Input: part model. Units: mm. Frame: model coordinates. A direction names the side the tool comes from. Round coordinates to 2 decimals unless told otherwise and drop trailing zeros. Loops run counter-clockwise (first coordinate to the right, second up) from the corner with the lowest first, then second, coordinate; pieces in that order, holes last. Notation, with made-up numbers: (79.5, 9.25) - (131.5, 9.25) arc R13 ccw to (131.5, 17.25) - close; hole circle Ø4 at (16, 3.25). An arc over 180 degrees is marked (long way). One line per question, with ' | ' between items. Start each with the question number.
from build123d import *

# Parameters (mm, degrees)
SKETCH1_W                = 100
SKETCH1_H                = 110
BOSS_EXTRUDE1_DEPTH      = 6.86
BOSS_EXTRUDE2_DEPTH      = 6.86
CUT_EXTRUDE1_DEPTH       = 84.419927529
CUT_EXTRUDE1_DEPTH_BACK  = 84.419927529
CUT_EXTRUDE5_DEPTH       = 84.419927529
CUT_EXTRUDE6_DEPTH       = 84.419927529
SKETCH7_W                = 42
SKETCH7_H                = 3.55
CUT_EXTRUDE7_DEPTH       = 84.419927529
SKETCH8_W                = 5
SKETCH8_H                = 7.62
CUT_EXTRUDE8_DEPTH       = 84.419927529
CUT_EXTRUDE9_DEPTH       = 84.419927529
LPATTERN1_COUNT          = 2
LPATTERN1_PITCH          = 49.4
SKETCH15_W               = 6.5
SKETCH15_H               = 9.5
BOSS_EXTRUDE3_DEPTH      = 6.86
CUT_EXTRUDE14_START      = -6.86
CUT_EXTRUDE14_DEPTH      = 6.86
BOSS_EXTRUDE4_DEPTH      = 6.86
FILLET3_R                = 5
FILLET4_R                = 7
CUT_EXTRUDE11_DEPTH      = 84.419927529
BOSS_EXTRUDE5_DEPTH      = 6.86
BOSS_EXTRUDE6_DEPTH      = 6.86
CUT_EXTRUDE12_DEPTH      = 84.419927529
CUT_EXTRUDE12_DEPTH_BACK = 84.419927529
SKETCH22_R               = 1
CUT_EXTRUDE13_DEPTH      = 84.419927529
CUT_EXTRUDE15_DEPTH      = 84.419927529
CUT_EXTRUDE15_DEPTH_BACK = 84.419927529
CUT_EXTRUDE16_DEPTH      = 84.419927529
CUT_EXTRUDE16_DEPTH_BACK = 84.419927529
FILLET2_R                = 1
BOSS_EXTRUDE8_START      = -6.86
BOSS_EXTRUDE8_DEPTH      = 6.86
CUT_EXTRUDE19_START      = -10
CUT_EXTRUDE19_DEPTH      = 10
SKETCH28_W               = 6.86
SKETCH28_H               = 9.5
SKETCH28_H_2             = 35
BOSS_EXTRUDE9_DEPTH      = 0.4
BOSS_EXTRUDE10_REACH     = 81.915
SKETCH29_W               = 6.86
SKETCH29_H               = 0.5
BOSS_EXTRUDE11_DEPTH     = 6.86


# Read off the part's stored shape, not the designer's step: Cut-Extrude14
with BuildPart() as part:
    # Sketch1 → Boss-Extrude1 (new body)
    with BuildSketch(Plane.XY):
        Rectangle(SKETCH1_W, SKETCH1_H)
    extrude(amount=BOSS_EXTRUDE1_DEPTH)

    # Sketch14 → Boss-Extrude2 (add)
    with BuildSketch(Plane.XY.offset(6.86)):
        with BuildLine():
            Line((-50, 44), (-56.9, 44))
            Line((-56.9, 44), (-57.252653961, 46))
            Line((-57.252653961, 46), (-60.252653961, 46))
            ThreePointArc((-60.252653961, 46), (-62.140394827, 27.177051725), (-56.9, 9))
            Line((-56.9, 9), (-50, 9))
            Line((-50, 9), (-50, 44))
        make_face()
    extrude(amount=-BOSS_EXTRUDE2_DEPTH)

    # Sketch9 → Cut-Extrude1 (cut, two sides: drawn at the far end of the back side and taken through both)
    with BuildSketch(Plane.XY.offset(6.86).offset(-CUT_EXTRUDE1_DEPTH_BACK)):
        Polygon((-202.691345573, 326.397371639), (-46, 55), (2.5, -29.004464167), (-49.825975731, -59.214880341), (-321.22334737, -215.906225914), (291.08659924, -349.739606366), (409.618601037, 192.563991188), align=None)
    extrude(amount=CUT_EXTRUDE1_DEPTH + CUT_EXTRUDE1_DEPTH_BACK, mode=Mode.SUBTRACT)

    # Sketch11 → Cut-Extrude5 (cut, through all)
    with BuildSketch(Plane.XY.offset(6.86)):
        Polygon((-35.90593882, 37.516573181), (-8.20593882, -10.461234188), (-15.13414205, -14.461234188), (-42.83414205, 33.516573181), align=None)
    extrude(amount=-CUT_EXTRUDE5_DEPTH, mode=Mode.SUBTRACT)

    # Sketch12 → Cut-Extrude6 (cut, through all)
    with BuildSketch(Plane.XY.offset(6.86)):
        Polygon((-18.88414205, -7.96604366), (-21.534179786, -9.49604366), (-35.534179786, 14.752667646), (-32.88414205, 16.282667646), align=None)
    extrude(amount=-CUT_EXTRUDE6_DEPTH, mode=Mode.SUBTRACT)

    # Sketch7 → Cut-Extrude7 (cut, through all)
    with BuildSketch(Plane.XY.offset(6.86)):
        with Locations((-50, -34)):
            Rectangle(SKETCH7_W, SKETCH7_H)
    extrude(amount=-CUT_EXTRUDE7_DEPTH, mode=Mode.SUBTRACT)

    # Sketch8 → Cut-Extrude8 (cut, through all)
    with BuildSketch(Plane.XY.offset(6.86)):
        with Locations((-36.5, -34)):
            Rectangle(SKETCH8_W, SKETCH8_H)
    extrude(amount=-CUT_EXTRUDE8_DEPTH, mode=Mode.SUBTRACT)

    # Sketch13 → Cut-Extrude9 (cut, through all)
    with BuildSketch(Plane.XY.offset(6.86)):
        Polygon((-41.88414205, 31.871124914), (-40.78414205, 29.965869026), (-48.578370684, 25.465869026), (-48.048870684, 24.548748123), (-49.478678626, 23.723248123), (-50.008178626, 24.640369026), (-52.908497703, 22.965869026), (-54.008497703, 24.871124914), (-51.108178626, 26.545624914), (-51.637678626, 27.462745817), (-50.207870684, 28.288245817), (-49.678370684, 27.371124914), align=None)
        Polygon((-39.45593882, 43.665353548), (-38.35593882, 41.76009766), (-46.150167454, 37.26009766), (-45.620667454, 36.342976757), (-47.050475396, 35.517476757), (-47.579975396, 36.43459766), (-50.480294473, 34.76009766), (-51.580294473, 36.665353548), (-48.679975396, 38.339853548), (-49.209475396, 39.256974451), (-47.779667454, 40.082474451), (-47.250167454, 39.165353548), align=None)
        Polygon((-18.443009001, -24.930108514), (-11.443009001, -37.054464167), (-9.537753113, -35.954464167), (-16.537753113, -23.830108514), align=None)
    cut_extrude9 = extrude(amount=-CUT_EXTRUDE9_DEPTH, mode=Mode.SUBTRACT)

    # LPattern1: Cut-Extrude9 ×2
    with Locations(*[Vector(0.49999999999999345, -0.8660254037844425, 0) * (i * LPATTERN1_PITCH) for i in range(1, LPATTERN1_COUNT)]):
        add(cut_extrude9, mode=Mode.SUBTRACT)

    # Sketch15 → Boss-Extrude3 (add)
    with BuildSketch(Plane.XY.offset(6.86)):
        with Locations((-53.25, -19.75)):
            Rectangle(SKETCH15_W, SKETCH15_H)
    extrude(amount=-BOSS_EXTRUDE3_DEPTH)

    # Cut-Extrude14 outline → Cut-Extrude14 (cut)
    with BuildSketch(Plane.XY.offset(6.86).offset(CUT_EXTRUDE14_START)):
        Polygon((-56.5, -15), (-56.5, -16.500643242), (-50, -15), align=None)
    extrude(amount=CUT_EXTRUDE14_DEPTH, mode=Mode.SUBTRACT)

    # Sketch16 → Boss-Extrude4 (add)
    with BuildSketch(Plane.XY.offset(6.86)):
        Polygon((-35.605117767, -51.004464167), (-34.105117767, -53.602540378), (-36.525588833, -55), (-42.525588833, -55), (-44.558274136, -51.479285778), align=None)
    extrude(amount=-BOSS_EXTRUDE4_DEPTH)

    # Fillet3
    fillet3_edges = [part.edges().sort_by_distance(p)[0] for p in [
        (2.5, -29.004464167, 3.43),
    ]]
    fillet(fillet3_edges, radius=FILLET3_R)

    # Fillet4
    fillet4_edges = [part.edges().sort_by_distance(p)[0] for p in [
        (-56.9, 9, 3.43),
    ]]
    fillet(fillet4_edges, radius=FILLET4_R)

    # Sketch18 → Cut-Extrude11 (cut, through all)
    with BuildSketch(Plane.XY.offset(6.86)):
        Polygon((-17.686495929, -28.360427591), (-13.945266185, -26.200427591), (-13.119766185, -27.630235533), (-16.860995929, -29.790235533), align=None)
    extrude(amount=-CUT_EXTRUDE11_DEPTH, mode=Mode.SUBTRACT)

    # Sketch19 → Boss-Extrude5 (add)
    with BuildSketch(Plane.XY.offset(6.86)):
        Polygon((-24.334179786, -4.646301399), (-23.234179786, -6.551557287), (-25.780294473, -8.021557287), (-26.880294473, -6.116301399), align=None)
    extrude(amount=-BOSS_EXTRUDE5_DEPTH)

    # Sketch20 → Boss-Extrude6 (add)
    with BuildSketch(Plane.XY.offset(6.86)):
        Polygon((-32.88414205, 16.282667646), (-18.88414205, -7.96604366), (-23.822038778, -10.816939665), (-37.822038778, 13.431771641), align=None)
    extrude(amount=-BOSS_EXTRUDE6_DEPTH)

    # Sketch21 → Cut-Extrude12 (cut, two sides: drawn at the far end of the back side and taken through both)
    with BuildSketch(Plane.XY.offset(6.86).offset(-CUT_EXTRUDE12_DEPTH_BACK)):
        Polygon((-50, 55), (-50, 44), (-48.060403212, 55), align=None)
    extrude(amount=CUT_EXTRUDE12_DEPTH + CUT_EXTRUDE12_DEPTH_BACK, mode=Mode.SUBTRACT)

    # Sketch22 → Cut-Extrude13 (cut, through all)
    with BuildSketch(Plane.XY.offset(6.86)):
        with Locations((-38, -5)):
            Circle(SKETCH22_R)
    extrude(amount=-CUT_EXTRUDE13_DEPTH, mode=Mode.SUBTRACT)

    # Sketch24 → Cut-Extrude15 (cut, two sides: drawn at the far end of the back side and taken through both)
    with BuildSketch(Plane.XY.offset(6.86).offset(-CUT_EXTRUDE15_DEPTH_BACK)):
        Polygon((207.425051562, 16.452548282), (-35.605117767, -51.004464167), (-50, -55), (-293.030169328, -122.457012449), (-158.11614443, -608.517351106), (342.33907646, -469.607790375), align=None)
    extrude(amount=CUT_EXTRUDE15_DEPTH + CUT_EXTRUDE15_DEPTH_BACK, mode=Mode.SUBTRACT)

    # Sketch26 → Cut-Extrude16 (cut, two sides: drawn at the far end of the back side and taken through both)
    with BuildSketch(Plane.XY.offset(6.86).offset(-CUT_EXTRUDE16_DEPTH_BACK)):
        Polygon((209.546353054, 0.01089), (-35.605117767, -51.004464167), (-50, -54), (-295.15147082, -105.015354167), (-193.120762486, -595.318295807), (311.577061387, -490.29205164), align=None)
    extrude(amount=CUT_EXTRUDE16_DEPTH + CUT_EXTRUDE16_DEPTH_BACK, mode=Mode.SUBTRACT)

    # Fillet2
    fillet2_edges = [part.edges().sort_by_distance(p)[0] for p in [
        (-60.252653961, 46, 3.43),
        (-56.5, -24.5, 3.43),
        (-56.5, -16.500643242, 3.43),
        (-50, -54, 3.43),
    ]]
    fillet(fillet2_edges, radius=FILLET2_R)

    # Sketch27 → Boss-Extrude8 (add)
    with BuildSketch(Plane.XY.offset(6.86).offset(BOSS_EXTRUDE8_START)):
        with BuildLine():
            Line((-55.724951054, -16.321709094), (-50, -15))
            Line((-50, -15), (-56.5, -15))
            Line((-56.5, -15), (-56.5, -17.296079159))
            ThreePointArc((-56.5, -17.296079159), (-56.282608157, -16.673564522), (-55.724951054, -16.321709094))
        make_face()
        with BuildLine():
            ThreePointArc((-52.380008746, 9), (-54.54635817, 9.343654894), (-56.5, 10.340877094))
            Line((-56.5, 10.340877094), (-56.5, 9))
            Line((-56.5, 9), (-52.380008746, 9))
        make_face()
        with BuildLine():
            Line((-56.5, -24.5), (-55.5, -24.5))
            ThreePointArc((-55.5, -24.5), (-56.207106781, -24.207106781), (-56.5, -23.5))
            Line((-56.5, -23.5), (-56.5, -24.5))
        make_face()
    extrude(amount=BOSS_EXTRUDE8_DEPTH)

    # Sketch27<5> → Cut-Extrude19 (cut)
    with BuildSketch(Plane.XY.offset(6.86).offset(CUT_EXTRUDE19_START)):
        with BuildLine():
            Line((-56.5, 10.340877094), (-56.5, 44))
            Line((-56.5, 44), (-56.9, 44))
            Line((-56.9, 44), (-57.252653961, 46))
            Line((-57.252653961, 46), (-59.50182182, 46))
            ThreePointArc((-59.50182182, 46), (-60.105291207, 45.797386167), (-60.464218102, 45.271649399))
            ThreePointArc((-60.464218102, 45.271649399), (-62.283923616, 29.230647449), (-58.897432775, 13.445947531))
            ThreePointArc((-58.897432775, 13.445947531), (-57.920678072, 11.722035132), (-56.5, 10.340877094))
        make_face()
    extrude(amount=CUT_EXTRUDE19_DEPTH, mode=Mode.SUBTRACT)

    # Sketch28 → Boss-Extrude9 (add)
    with BuildSketch(Plane.ZY.offset(56.5)):
        with Locations((3.43, -19.75)):
            Rectangle(SKETCH28_W, SKETCH28_H)
        with Locations((3.43, 26.5)):
            Rectangle(SKETCH28_W, SKETCH28_H_2)
    extrude(amount=BOSS_EXTRUDE9_DEPTH)

    # Sketch29 → Boss-Extrude10 (add, up to next)
    with BuildSketch(Plane.ZY.offset(56.9), mode=Mode.PRIVATE) as boss_extrude10_sk1:
        with Locations((3.43, -14.75)):
            Rectangle(SKETCH29_W, SKETCH29_H)
    boss_extrude10_tool1 = extrude(boss_extrude10_sk1.sketch, amount=-BOSS_EXTRUDE10_REACH, mode=Mode.PRIVATE) - part.part
    add(boss_extrude10_tool1.solids().sort_by_distance((-56.9, -14.75, 3.43))[0])

    # Sketch30 → Boss-Extrude11 (add)
    with BuildSketch(Plane.XY.offset(6.86)):
        Polygon((-39, -32.225), (-50, -32.225), (-50, -35.775), (-39, -35.775), (-39, -37.81), (-34, -37.81), (-34, -35.775), (-29, -35.775), (-29, -32.225), (-34, -32.225), (-34, -30.19), (-39, -30.19), align=None)
        Polygon((-50, 55), (-48.060403212, 55), (-50, 44), align=None)
    extrude(amount=-BOSS_EXTRUDE11_DEPTH)


solid = part.part
(1) Pin query (flat end, axial travel): P1, Ø1, axis at x = -6.5, z = 2, coming from the -Y side; P2, Ø2, axis at x = -54.5, z = 4.5, coming from the +Y side; P3, Ø4, axis at x = -28, z = 5.5, coming from the +Y side. Return the tip coordinate at first contact, or that it passes through.
(2) Pull-direction query (X, two-part tool) for faces 3 (the face through (-39.4, 35.5, 3.5)), 4 (the face through (-53.451, 23.905, 3.478)), 5 (the face through (-56.9, 27, 3)); classes: released by +X, released by -X, zero draft, split by the parting line, or undercut.
(3) Reachability of faces 1 (the face through (-42.774, 49.412, 3.382)), 2 (the face through (-45.836, 29.59, 3.478)) from +Z, -Z, +X, -X, +Y, -Y: full face, straight path, thin tool, end or side. Return the list, or none.
(4) Section C-C, the plane y = 19. Output: boundary loops of the cut face in (x, z).
(5) Line query: line 1 along Y through (x, z) = (-38, 2.75); line 2 along Y through (x, z) = (-40.5, 3.25); line 3 along Y through (x, z) = (-48.5, 4). Output: solid intervals per line, ascending. Write a range as from..to.
(6) Section A-A, the plane x = -44. Output: boundary loops of the cut face in (y, z).
(7) Section D-D, the plane y = 6.5. Output: boundary loops of the cut face in (x, z), plus the area to 3 significant figures.
(8) Section B-B, the plane y = -5. Output: boundary loops of the cut face in (x, z), plus the area to 3 significant figures.
Derived:
1) P1: stops at y = -34.49 | P2: stops at y = 44 | P3: stops at y = 11.29
2) face 3: released by +X | face 4: undercut | face 5: released by -X
3) face 1: +Z, -Z, +X, +Y | face 2: +Z, -Z
4) outline: (-56.9, 0) - (-34.45, 0) - (-34.45, 6.86) - (-56.9, 6.86) - close
5) line 1: y = -51.5..-6, -4..25.14, 36.31..41.14 | line 2: y = -52.02..29.47, 34.86..40.52, 43.06..45.47 | line 3: y = -53.69..24.29, 25.33..25.51, 28.05..35.9, 39.67..55
6) outline: (-52.75, 0) - (28.11, 0) - (28.11, 6.86) - (-52.75, 6.86) - close; (30.65, 0) - (38.5, 0) - (38.5, 6.86) - (30.65, 6.86) - close; (41.04, 0) - (51.54, 0) - (51.54, 6.86) - (41.04, 6.86) - close
7) outline: (-50, 0) - (-27.24, 0) - (-27.24, 6.86) - (-50, 6.86) - close | area: 156 mm²
8) outline: (-50, 0) - (-39, 0) - (-39, 6.86) - (-50, 6.86) - close; (-37, 0) - (-20.6, 0) - (-20.6, 6.86) - (-37, 6.86) - close | area: 188 mm²
